Drawing for the job (mm, zero at the part's lowest x, y, z). Coordinates: 2 decimals unless noted, no trailing zeros. Order: outer loops, then holes, each group sorted by start corner. A loop starts at its lowest first (then second) coordinate and runs counter-clockwise, first axis right, second up. Notation, with made-up numbers: (38.25, 4) - (61.25, 4) arc R25 cw to (61.25, 34) - close; hole circle Ø4 at (25, 64.5). An arc over 180 degrees is marked (long way). Put each result on its own line as item: value. Start each with the question number.
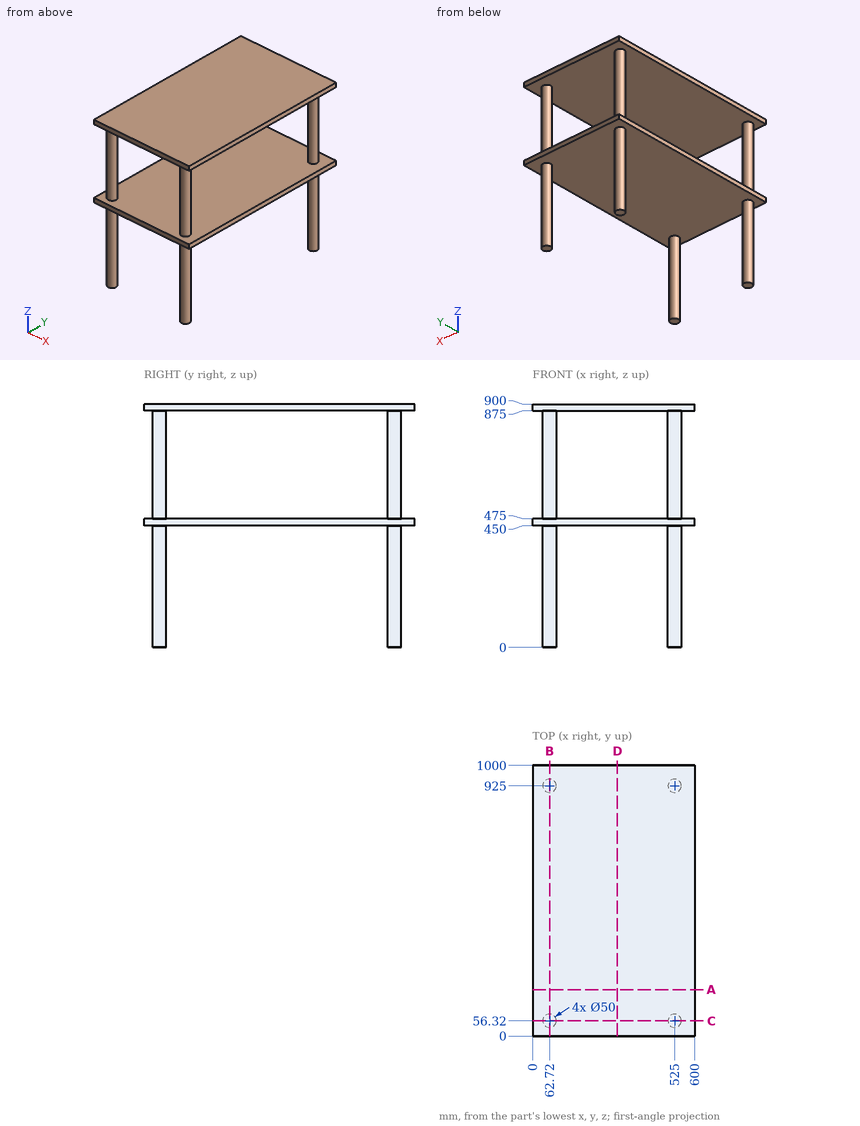
Item 1: Slice it at C-C, the plane y = 56.32. Give the cut face in (x, z), plus the area to 3 significant figures.
Item 2: Slice it at D-D, the plane x = 313. Give the cut face in (y, z).
Item 3: Wall check: line 1 along Z through (x, y) = (363, 52.5); line 2 along Y through (x, z) = (77, 703); line 3 along X through (y, z) = (65, 512). Give the ranges that are in metal, low to high.
Item 4: Slice it at A-A, the plane y = 171.5. Give the cut face in (x, z), plus the area to 3 significant figures.
Item 5: Flat gauge pins, fed straight in: pin 1 Ø12 at (x, y) = (259, 502) entering from -Z; pin 2 Ø2 at (x, z) = (527.5, 251) entering from -Y. Where does each tip first touch, or does it go through?
Item 6: Slice it at B-B, the plane x = 62.72. Give the cut face in (y, z).
Here are the results:
1. outline: (0, 450) - (37.72, 450) - (37.72, 0) - (87.72, 0) - (87.72, 450) - (500, 450) - (500, 0) - (550, 0) - (550, 450) - (600, 450) - (600, 475) - (550, 475) - (550, 875) - (600, 875) - (600, 900) - (0, 900) - (0, 875) - (37.72, 875) - (37.72, 475) - (0, 475) - close; hole (87.72, 475) - (500, 475) - (500, 875) - (87.72, 875) - close
1. area: 115,000 mm^2
2. outline: (0, 450) - (1000, 450) - (1000, 475) - (0, 475) - close; (0, 875) - (1000, 875) - (1000, 900) - (0, 900) - close
3. line 1: z = 450 to 475, 875 to 900
3. line 2: y = 35.8 to 76.84, 904.48 to 945.52
3. line 3: x = 39.28 to 86.16, 501.56 to 548.44
4. outline: (0, 450) - (600, 450) - (600, 475) - (0, 475) - close; (0, 875) - (600, 875) - (600, 900) - (0, 900) - close
4. area: 30,000 mm^2
5. pin 1: stops at z = 450
5. pin 2: stops at y = 31.37
6. outline: (0, 450) - (31.32, 450) - (31.32, 0) - (81.32, 0) - (81.32, 450) - (900, 450) - (900, 0) - (950, 0) - (950, 450) - (1000, 450) - (1000, 475) - (950, 475) - (950, 875) - (1000, 875) - (1000, 900) - (0, 900) - (0, 875) - (31.32, 875) - (31.32, 475) - (0, 475) - close; hole (81.32, 475) - (900, 475) - (900, 875) - (81.32, 875) - close
